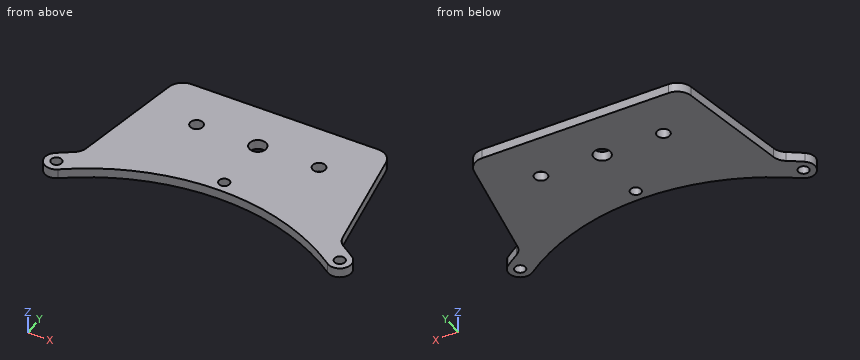
from build123d import *

# Parameters (mm, degrees)
SKETCH1_R           = 1.75
SKETCH1_R_2         = 2.1
SKETCH1_R_3         = 2.75
BOSS_EXTRUDE1_DEPTH = 1.5875


with BuildPart() as part:
    # Sketch1 → Boss-Extrude1 (new, symmetric)
    with BuildSketch(Plane.XY):
        with BuildLine():
            Line((-30.5, 34.81), (30.5, 34.81))
            ThreePointArc((30.5, 34.81), (33.713938048, 33.640222216), (35.424038765, 30.678240888))
            Line((35.424038765, 30.678240888), (41.817257659, -5.579505193))
            ThreePointArc((41.817257659, -5.579505193), (42.58957924, -7.49752424), (44.071890575, -8.939061889))
            ThreePointArc((44.071890575, -8.939061889), (46.321344226, -10.411121997), (48.521672577, -11.955647114))
            ThreePointArc((48.521672577, -11.955647114), (49.364565514, -17.277463674), (44.042748954, -18.120356611))
            ThreePointArc((44.042748954, -18.120356611), (0, -3.81), (-44.042748954, -18.120356611))
            ThreePointArc((-44.042748954, -18.120356611), (-49.364565514, -17.277463674), (-48.521672577, -11.955647114))
            ThreePointArc((-48.521672577, -11.955647114), (-46.321344226, -10.411121997), (-44.071890575, -8.939061889))
            ThreePointArc((-44.071890575, -8.939061889), (-42.58957924, -7.49752424), (-41.817257659, -5.579505193))
            Line((-41.817257659, -5.579505193), (-35.424038765, 30.678240888))
            ThreePointArc((-35.424038765, 30.678240888), (-33.713938048, 33.640222216), (-30.5, 34.81))
        make_face()
        Circle(SKETCH1_R, mode=Mode.SUBTRACT)
        with Locations((-46.282210766, -15.038001863)):
            Circle(SKETCH1_R, mode=Mode.SUBTRACT)
        with Locations((46.282210766, -15.038001863)):
            Circle(SKETCH1_R, mode=Mode.SUBTRACT)
        with Locations((-20, 19.31)):
            Circle(SKETCH1_R_2, mode=Mode.SUBTRACT)
        with Locations((20, 19.31)):
            Circle(SKETCH1_R_2, mode=Mode.SUBTRACT)
        with Locations((0, 19.31)):
            Circle(SKETCH1_R_3, mode=Mode.SUBTRACT)
    extrude(amount=BOSS_EXTRUDE1_DEPTH, both=True)


solid = part.part
CAD build for the part. Positions are in the model's coordinates, mm. Round coordinates to 2 decimals unless told otherwise and drop trailing zeros. Write each loop counter-clockwise with the first axis right and the second up, starting at its lowest first coordinate (ties: lowest second). Pieces come first, ordered by that corner, then holes. Notation, with made-up numbers: M 42.5,10 L 100.5,10 A14 ccw 100.5,22 Z; hole C 17.25,80 d3. An arc over 180 degrees is marked long. Use a Markdown table: item, result. Add a question column.
1. Drill centre lines: probe 1 along Y at (x, z) = (0, 0.1); probe 2 along Y at (x, z) = (-0.5, -0.2); probe 3 along X at (y, z) = (17, -0.3). Where is each one in solid material? Low to high.
2. Slice it at D-D on y = 19.31. Give the cut face in (x, z).
3. Slice it at B-B on y = 0. Give the cut face in (x, z), then the cut area to 3 significant figures.
4. Slice it at C-C on x = -20. Give the cut face in (y, z).
5. Flat gauge pin, fed straight in: P1, Ø1.5, axis at x = 5, z = -1, coming from the -Y side. Where does the tip first touch, or does it go through?
6. Slice it at A-A on z = 0.05. Give the cut face in (x, y).
Reply:
| question | item | result |
|---|---|---|
| 1 | probe 1 | y = -3.81 to -1.75, 1.75 to 16.56, 22.06 to 34.81 |
| 1 | probe 2 | y = -3.81 to -1.68, 1.68 to 16.61, 22.01 to 34.81 |
| 1 | probe 3 | x = -37.84 to -1.49, 1.49 to 37.84 |
| 2 | outline | M -37.43,-1.59 L -22.1,-1.59 L -22.1,1.59 L -37.43,1.59 Z; M -17.9,-1.59 L -2.75,-1.59 L -2.75,1.59 L -17.9,1.59 Z; M 2.75,-1.59 L 17.9,-1.59 L 17.9,1.59 L 2.75,1.59 Z; M 22.1,-1.59 L 37.43,-1.59 L 37.43,1.59 L 22.1,1.59 Z |
| 3 | outline | M -40.83,-1.59 L -1.75,-1.59 L -1.75,1.59 L -40.83,1.59 Z; M 1.75,-1.59 L 40.83,-1.59 L 40.83,1.59 L 1.75,1.59 Z |
| 3 | area | 248 mm^2 |
| 4 | outline | M -6.53,-1.59 L 17.21,-1.59 L 17.21,1.59 L -6.53,1.59 Z; M 21.41,-1.59 L 34.81,-1.59 L 34.81,1.59 L 21.41,1.59 Z |
| 5 | P1 | stops at y = -4.03 |
| 6 | outline | M -48.52,-11.96 A3.81 ccw -44.04,-18.12 A74.93 cw 44.04,-18.12 A3.81 ccw 48.52,-11.96 A82.55 ccw 44.07,-8.94 A5 cw 41.82,-5.58 L 35.42,30.68 A5 ccw 30.5,34.81 L -30.5,34.81 A5 ccw -35.42,30.68 L -41.82,-5.58 A5 cw -44.07,-8.94 A82.55 ccw Z; hole C -46.28,-15.04 d3.5; hole C -20,19.31 d4.2; hole C 0,19.31 d5.5; hole C 0,0 d3.5; hole C 20,19.31 d4.2; hole C 46.28,-15.04 d3.5 |
